Could you check a few things on this model? Use its own coordinates, in mm. Face numbers are marked on the shaded views. A direction names the side the tool comes from. Coordinates: 2 decimals unless noted, no trailing zeros. Order: outer loops, then holes, each group sorted by start corner. A loop starts at its lowest first (then second) coordinate and runs counter-clockwise, first axis right, second up. Notation, with made-up numbers: (37, 60.5) - (53, 60.5) arc R18 ccw to (53, 76.5) - close; hole circle Ø7 at (35.5, -26.5). An arc over 180 degrees is marked (long way). One line per item, written item: value. Start each with the question number.
from build123d import *

# Parameters (mm, degrees)
SKETCH1_W           = 30
SKETCH1_H           = 25
BOSS_EXTRUDE1_DEPTH = 25
CUT_EXTRUDE1_DEPTH  = 10
SKETCH3_W           = 10
SKETCH3_H           = 25
CUT_EXTRUDE3_DEPTH  = 10
SKETCH5_W           = 10
SKETCH5_H           = 15
CUT_EXTRUDE4_DEPTH  = 30
SKETCH6_W           = 10
SKETCH6_H           = 15
CUT_EXTRUDE5_DEPTH  = 10


with BuildPart() as part:
    # Sketch1 → Boss-Extrude1 (new body)
    with BuildSketch(Plane.XY):
        with Locations((15, 12.5)):
            Rectangle(SKETCH1_W, SKETCH1_H)
    extrude(amount=BOSS_EXTRUDE1_DEPTH)

    # Sketch2 → Cut-Extrude1 (cut)
    with BuildSketch(Plane.ZY):
        Polygon((0, 15), (5, 25), (0, 25), align=None)
        Polygon((25, 25), (20, 25), (25, 15), align=None)
    extrude(amount=-CUT_EXTRUDE1_DEPTH, mode=Mode.SUBTRACT)

    # Sketch3 → Cut-Extrude3 (cut)
    with BuildSketch(Plane(origin=(0, 25, 0), x_dir=(1, 0, 0), z_dir=(0, 1, 0))):
        with Locations((15, -12.5)):
            Rectangle(SKETCH3_W, SKETCH3_H)
    extrude(amount=-CUT_EXTRUDE3_DEPTH, mode=Mode.SUBTRACT)

    # Sketch5 → Cut-Extrude4 (cut)
    with BuildSketch(Plane(origin=(0, 15, 0), x_dir=(1, 0, 0), z_dir=(0, 1, 0))):
        with Locations((15, -12.5)):
            Rectangle(SKETCH5_W, SKETCH5_H)
    extrude(amount=-CUT_EXTRUDE4_DEPTH, mode=Mode.SUBTRACT)

    # Sketch6 → Cut-Extrude5 (cut)
    with BuildSketch(Plane(origin=(0, 25, 0), x_dir=(1, 0, 0), z_dir=(0, 1, 0))):
        with Locations((25, -12.5)):
            Rectangle(SKETCH6_W, SKETCH6_H)
    extrude(amount=-CUT_EXTRUDE5_DEPTH, mode=Mode.SUBTRACT)


solid = part.part
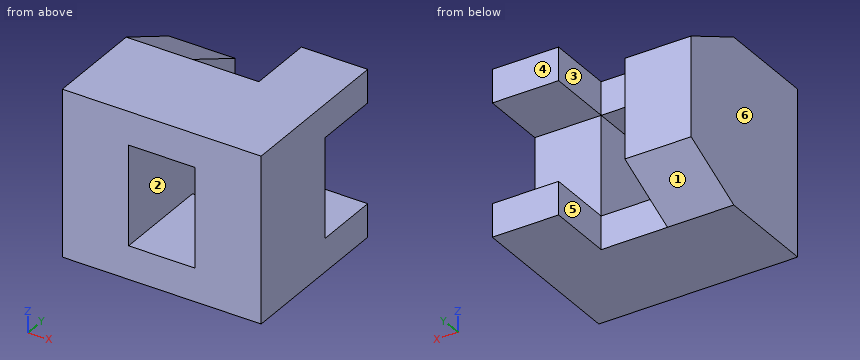
Q1. If I drill on L1, parallel to Z at x = 19, y = 5; L2, parallel to X at y = 9, z = 8.25; L3, parallel to X at y = 18.75, z = 8.75, over which ranges is the centre line in solid material (lowest first)?
Q2. I want a section at B-B on y = 17. Please give me the cut outline in (x, z), then the cut area to 3 significant figures.
Q3. Which directions (+Z, -Z, +X, -X, +Y, -Y) give clear straight access to the entire face, cutting with the end or side of a thin tool? Please do the marked faces 1, 2 and 3.
Q4. I want a section at D-D on y = 8.75. Please give me the cut outline in (x, z), then the cut area to 3 significant figures.
Q5. I want a section at A-A on z = 9. Please give me the cut outline in (x, y), then the cut area to 3 significant figures.
Q6. I'm going to push a flat-ended pin straight in: pin 1 (8 mm diameter, centred on x = 23.5, z = 12.5, fed in from +Y). Where does the tip first touch, or does it pass through?
Q7. I want a section at C-C on x = 14. Please give me the cut outline in (y, z), then the cut area to 3 significant figures.
Q8. We'd pull the mould along X, two halves only. Please class the marked faces 4, 5 and 6: +X half, -X half, draft (parallel to the pull), parting line (faces both ways), or undercut.
Values follow:
1. L1: z = 0 to 5, 20 to 25
1. L2: x = 0 to 10, 20 to 30
1. L3: x = 0 to 10
2. outline: (0, 1) - (10, 1) - (10, 24) - (0, 24) - close; (20, 0) - (30, 0) - (30, 5) - (20, 5) - close; (20, 20) - (30, 20) - (30, 25) - (20, 25) - close
2. area: 330 mm^2
3. face 1: -Z, -X, +Y
3. face 2: +Y
3. face 3: +Z, -Z, +Y
4. outline: (0, 0) - (30, 0) - (30, 25) - (0, 25) - close; hole (10, 5) - (20, 5) - (20, 20) - (10, 20) - close
4. area: 600 mm^2
5. outline: (0, 0) - (10, 0) - (10, 25) - (0, 25) - close; (20, 0) - (30, 0) - (30, 15) - (20, 15) - close
5. area: 400 mm^2
6. pin 1: stops at y = 15
7. outline: (0, 0) - (15, 0) - (15, 5) - (0, 5) - close; (0, 20) - (15, 20) - (15, 25) - (0, 25) - close
7. area: 150 mm^2
8. face 4: draft
8. face 5: undercut
8. face 6: -X half
